```python
from build123d import *

# Parameters (mm, degrees)
SKETCH1_R           = 4
BOSS_EXTRUDE1_DEPTH = 22
SKETCH2_R           = 4
BOSS_EXTRUDE2_DEPTH = 17
BOSS_EXTRUDE2_TAPER = 2.75
SKETCH3_R           = 2.786556444
BOSS_EXTRUDE3_DEPTH = 8


with BuildPart() as part:
    # Sketch1 → Boss-Extrude1 (new body)
    with BuildSketch(Plane(origin=(0, 0, 0), x_dir=(1, 0, 0), z_dir=(0, 1, 0))):
        with Locations(Location((0, 0, 0), (0, 0, 270))):
            Circle(SKETCH1_R)
    extrude(amount=BOSS_EXTRUDE1_DEPTH)

    # Sketch2 → Boss-Extrude2 (add)
    with BuildSketch(Plane(origin=(0, 22, 0), x_dir=(1, 0, 0), z_dir=(0, 1, 0))):
        with Locations(Location((0, 0, 0), (0, 0, 270))):
            Circle(SKETCH2_R)
    extrude(amount=BOSS_EXTRUDE2_DEPTH, taper=BOSS_EXTRUDE2_TAPER)

    # Sketch3 → Boss-Extrude3 (add)
    with BuildSketch(Plane(origin=(0, 39, 0), x_dir=(1, 0, 0), z_dir=(0, 1, 0))):
        with Locations(Location((0, 0, 0), (0, 0, 270))):
            Circle(SKETCH3_R)
    extrude(amount=BOSS_EXTRUDE3_DEPTH)


solid = part.part
```
Source: CAD feature listing. Evaluate the final solid. Frame: model axes, mm. A direction names the side the tool comes from. Coordinates: 2 decimals unless noted, no trailing zeros. Loops run counter-clockwise (first coordinate to the right, second up) from the corner with the lowest first, then second, coordinate; pieces in that order, holes last. Notation, with made-up numbers: M 84.5,7.25 L 132.5,7.25 A24 cw 132.5,21.25 Z; hole C -3,-20 d10. An arc over 180 degrees is marked long. Use CSV: the item, a comma, the result in double quotes.
(1) Contact query for flat-ended pins moving along their axis: pin 1 (3 mm diameter, centred on x = 2, y = 42, fed in from +Z); pin 2 (1.5 mm diameter, centred on y = 25, z = 0.5, fed in from -X). Output: stop coordinate, or through.
Answers follow:
pin 1,"z = 2.74"
pin 2,"x = -3.89"
(2) Cut plane B-B on y = 33.5. Return loops of the section in (x, z), and give its area (3 significant figures).
Answers follow:
outline,"C 0,0 d6.9"
area,"37.3 mm²"
(3) Line query: line 1 (Y direction, x = 1.5, z = -2.75); line 2 (X direction, y = 5, z = -2.5); line 3 (Z direction, x = -2, y = 12.5). Output: solid intervals per line, ascending. Write a range as [from, to].
Answers follow:
line 1,"[0, 39]"
line 2,"[-3.12, 3.12]"
line 3,"[-3.46, 3.46]"
(4) Reachability of faces 1 (the face through (-3.905, 10.846, -0.867)), 2 (the face through (-3, 39, 0)) from +Z, -Z, +X, -X, +Y, -Y: full face, straight path, thin tool, end or side. Return the list, or none.
Answers follow:
face 1,"+Y, -Y"
face 2,"+Y"
(5) Cut plane A-A on z = 0. Return loops of the section in (x, y), and give its area (3 significant figures).
Answers follow:
outline,"M -4,0 L 4,0 L 4,22 L 3.18,39 L 2.79,39 L 2.79,47 L -2.79,47 L -2.79,39 L -3.18,39 L -4,22 Z"
area,"343 mm²"
(6) Cut plane C-C on y = 12. Return loops of the section in (x, z).
Answers follow:
outline,"C 0,0 d8"
